from build123d import *

# Parameters (mm, degrees)
F4_DEPTH  = 7.5
F7_DEPTH  = 9
F8_DEPTH  = 14.001
F9_W      = 61.8011951447
F9_H      = 108.7959855795
F9_W_2    = 52.8042912483
F9_H_2    = 139.1329020262
F10_DEPTH = 42.5010001
F11_DEPTH = 42.5010001
F12_SIZE  = 2


with BuildPart() as f1:
    # F0 (on Front) → F1 (revolve)
    with BuildSketch(Plane.XZ):
        Polygon((-291, 35), (-291, 0), (291, 0), (291, 35), (151, 35), (151, 37.5), (99, 37.5), (99, 42.5), (63, 42.5), (63, 37.5), (-16, 37.5), (-16, 37.3), (-98, 37.3), (-98, 37.5), (-151, 37.5), (-151, 35), align=None)
    revolve(axis=Axis((0, 0, 0), (-1, 0, 0)))

    # F3 (on offset) → F4 (cut)
    with BuildSketch(Plane.XY.offset(35)):
        with BuildLine():
            Line((-168.5, 10), (-273.5, 10))
            ThreePointArc((-273.5, 10), (-266.4289321881, 7.0710678119), (-263.5, 0))
            ThreePointArc((-263.5, 0), (-266.4289321881, -7.0710678119), (-273.5, -10))
            Line((-273.5, -10), (-168.5, -10))
            ThreePointArc((-168.5, -10), (-178.5, 0), (-168.5, 10))
        make_face()
        with BuildLine():
            ThreePointArc((-263.5, 0), (-266.4289321881, 7.0710678119), (-273.5, 10))
            Line((-273.5, 10), (-273.5, -10))
            ThreePointArc((-273.5, -10), (-266.4289321881, -7.0710678119), (-263.5, 0))
        make_face()
        with BuildLine():
            Line((-273.5, -10), (-273.5, 10))
            ThreePointArc((-273.5, 10), (-283.5, 0), (-273.5, -10))
        make_face()
        with BuildLine():
            Line((-168.5, -10), (-168.5, 10))
            ThreePointArc((-168.5, 10), (-178.5, 0), (-168.5, -10))
        make_face()
        with BuildLine():
            ThreePointArc((-158.5, 0), (-161.4289321881, 7.0710678119), (-168.5, 10))
            Line((-168.5, 10), (-168.5, -10))
            ThreePointArc((-168.5, -10), (-161.4289321881, -7.0710678119), (-158.5, 0))
        make_face()
        with BuildLine():
            Line((168.5, -10), (168.5, 10))
            ThreePointArc((168.5, 10), (158.5, 0), (168.5, -10))
        make_face()
        with BuildLine():
            ThreePointArc((178.5, 0), (175.5710678119, 7.0710678119), (168.5, 10))
            Line((168.5, 10), (168.5, -10))
            ThreePointArc((168.5, -10), (175.5710678119, -7.0710678119), (178.5, 0))
        make_face()
        with BuildLine():
            Line((273.5, -10), (273.5, 10))
            ThreePointArc((273.5, 10), (263.5, 0), (273.5, -10))
        make_face()
        with BuildLine():
            ThreePointArc((283.5, 0), (280.5710678119, 7.0710678119), (273.5, 10))
            Line((273.5, 10), (273.5, -10))
            ThreePointArc((273.5, -10), (280.5710678119, -7.0710678119), (283.5, 0))
        make_face()
        with BuildLine():
            Line((273.5, 10), (168.5, 10))
            ThreePointArc((168.5, 10), (175.5710678119, 7.0710678119), (178.5, 0))
            ThreePointArc((178.5, 0), (175.5710678119, -7.0710678119), (168.5, -10))
            Line((168.5, -10), (273.5, -10))
            ThreePointArc((273.5, -10), (263.5, 0), (273.5, 10))
        make_face()
    extrude(amount=-F4_DEPTH, mode=Mode.SUBTRACT)

    # F6 (on offset) → F7 (cut)
    with BuildSketch(Plane.XY.offset(37.5)):
        with BuildLine():
            ThreePointArc((73.1, 0), (69.8781745931, 7.7781745931), (62.1, 11))
            Line((62.1, 11), (62.1, -11))
            ThreePointArc((62.1, -11), (69.8781745931, -7.7781745931), (73.1, 0))
        make_face()
        with BuildLine():
            Line((62.1, 11), (-17.9, 11))
            ThreePointArc((-17.9, 11), (-10.1218254069, 7.7781745931), (-6.9, 0))
            ThreePointArc((-6.9, 0), (-10.1218254069, -7.7781745931), (-17.9, -11))
            Line((-17.9, -11), (62.1, -11))
            ThreePointArc((62.1, -11), (51.1, 0), (62.1, 11))
        make_face()
        with BuildLine():
            Line((62.1, -11), (62.1, 11))
            ThreePointArc((62.1, 11), (51.1, 0), (62.1, -11))
        make_face()
        with BuildLine():
            Line((-17.9, -11), (-17.9, 11))
            ThreePointArc((-17.9, 11), (-28.9, 0), (-17.9, -11))
        make_face()
        with BuildLine():
            ThreePointArc((-6.9, 0), (-10.1218254069, 7.7781745931), (-17.9, 11))
            Line((-17.9, 11), (-17.9, -11))
            ThreePointArc((-17.9, -11), (-10.1218254069, -7.7781745931), (-6.9, 0))
        make_face()
    extrude(amount=-F7_DEPTH, mode=Mode.SUBTRACT)

    # F8 (cut, through all): a face of the model
    f8_faces = [f1.faces().sort_by_distance(p)[0] for p in [
        (22.1, 0, 28.5),
    ]]
    extrude(f8_faces, amount=F8_DEPTH, mode=Mode.SUBTRACT)

    # F9 (on Top) → F10 (cut, through all)
    with BuildSketch(Plane.XY):
        with Locations((-300.9005975723, 0)):
            Rectangle(F9_W, F9_H)
        with Locations((296.4021456242, 0)):
            Rectangle(F9_W_2, F9_H_2)
    extrude(amount=-F10_DEPTH, mode=Mode.SUBTRACT)

    # F11 (cut, through all): faces of the model
    f11_faces = [f1.faces().sort_by_distance(p)[0] for p in [
        (-280.5, 0, 0),
        (280.5, 0, 0),
    ]]
    extrude(f11_faces, amount=-F11_DEPTH, mode=Mode.SUBTRACT)

    # F12
    f12_edges = [f1.edges().sort_by_distance(p)[0] for p in [
        (-270, 0, -35),
        (270, 0, -35),
    ]]
    chamfer(f12_edges, length=F12_SIZE)


solid = f1.part
Here's how the part is built. I have some questions about the finished solid (model axes, mm). A direction names the side the tool comes from. Coordinates: 2 decimals unless noted, no trailing zeros. Order: outer loops, then holes, each group sorted by start corner. A loop starts at its lowest first (then second) coordinate and runs counter-clockwise, first axis right, second up. Notation, with made-up numbers: (-6.75, 19.25) -> (36.25, 19.25) arc R9 cw to (36.25, 33.25) -> close; hole circle Ø2 at (34.5, 1.5). An arc over 180 degrees is marked (long way). Answer in a Markdown table with one row per item.
(1) Will these pins go through, and if not, where does the flat tip stop? pin 1 Ø1.5 at (x, z) = (91.5, -12.5) entering from +Y; pin 2 Ø1.5 at (x, z) = (169.5, 0) entering from +Y; pin 3 Ø3 at (x, z) = (-189.5, -22) entering from -Y.
Answer key:
| item | result |
|---|---|
| pin 1 | y = 40.84 |
| pin 2 | y = 35 |
| pin 3 | y = -28.37 |
(2) On a 3-axis mill with a long thin cutter (end or side, diameter ignored), from which of +Z, -Z, +X, -X, +Y, -Y can I reach the whole of each face in a straight line? I mean faces 1 (the face through (158.5, 0.2, 31.3)), 2 (the face through (209, -21, -28)), 3 (the face through (63, 29, -26)). Say none if no direction works.
Answer key:
| item | result |
|---|---|
| face 1 | +Z, +X |
| face 2 | +X |
| face 3 | -X |
(3) Please list where these lines run through material, in increasing order: probe 1 along Y at (x, z) = (97, -3); probe 2 along X at (y, z) = (-4.5, -35); probe 3 along Y at (x, z) = (148.5, 3).
Answer key:
| item | result |
|---|---|
| probe 1 | -42.39 to 42.39 |
| probe 2 | -151 to 151 |
| probe 3 | -37.38 to 37.38 |
(4) I want a section at A-A on x = 175. List the corners of the cut face in (y, z) for me, then the cut area to 3 significant figures.
Answer key:
| item | result |
|---|---|
| outline | (-10, 27.5) -> (-10, 33.54) arc R35 ccw (long way) to (10, 33.54) -> (10, 27.5) -> close |
| area | 3,710 mm^2 |
(5) I want a section at B-B on x = -125. List the corners of the cut face in (y, z) for me.
Answer key:
| item | result |
|---|---|
| outline | circle Ø75 at (0, 0) |
